Work out the finished part from the listing and answer in its coordinate system (mm). Round coordinates to 2 decimals unless told otherwise and drop trailing zeros. Order: outer loops, then holes, each group sorted by start corner. A loop starts at its lowest first (then second) coordinate and runs counter-clockwise, first axis right, second up. Notation, with made-up numbers: (89, -26.75) -> (128, -26.75) arc R23 cw to (128, 2.25) -> close; hole circle Ø11 at (70.25, 8). An arc over 180 degrees is marked (long way). Use a Markdown table: item, result. Add a question column.
Item 1: Flat-ended cylindrical pins translate along their axes: P1, Ø5, axis at y = -73, z = -9.5, coming from the +X side; P2, Ø2, axis at x = 0.5, z = -38.5, coming from the -Y side; P3, Ø2, axis at x = 2, y = -4.5, coming from the +Z side; P4, Ø4, axis at y = -60, z = -57.5, coming from the -X side. Find the tip coordinate at first contact, or state that the pin passes through.
Item 2: A cutting plane is placed at A-A, the plane y = -55. Determine the outline of the cut face in (x, z).
Item 3: A cutting plane is placed at D-D, the plane y = -72. Determine the outline of the cut face in (x, z), plus the area to 3 significant figures.
Item 4: A cutting plane is placed at C-C, the plane z = -47.9. Determine the outline of the cut face in (x, y) (3 decimals), plus the area to 3 significant figures.
Item 5: A cutting plane is placed at B-B, the plane x = 6. Determine the outline of the cut face in (y, z) (3 decimals), plus the area to 3 significant figures.
Item 6: Find the intervals of material crossed by L1, parallel to Z at x = 4.5, y = -12; L2, parallel to Y at x = 5, z = -47.9 (3 decimals); L3, parallel to Z at x = 7.75, y = -7 (3 decimals), in increasing order. Write a range as [from, to].
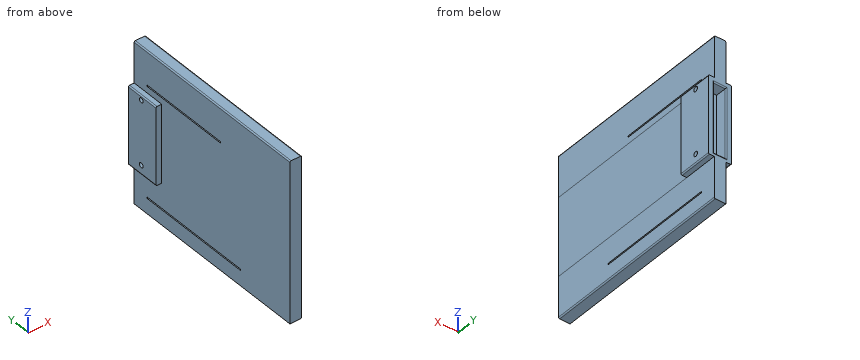
Autodesk Inventor part; units mm, degrees
ref_plane "YZ Plane" through (0, 0, 0) normal (1, 0, 0) x (0, 1, 0)
ref_plane "XZ Plane" through (0, 0, 0) normal (0, 1, 0) x (-1, 0, 0)
ref_plane "XY Plane" through (0, 0, 0) normal (0, 0, 1) x (1, 0, 0)
sketch "Sketch1" plane through (0, 0, 0) normal (1, 0, 0) x (0, 1, 0)
  line L0 (0, 0) -> (0, -70)
  line L1 (0, -70) -> (-85, -70)
  line L2 (-85, -70) -> (-85, 0)
  line L3 (-85, 0) -> (0, 0)
  dimension "d0" = 70
  dimension "d1" = 85
extrude "Extrusion1" add sketch "Sketch1" along normal blind 10
sketch "Sketch2" plane through (0, 0, 0) normal (0, 1, 0) x (1, 0, 0)
  line L0 (0, 0) -> (0, 70)
  line L1 (0, 0) -> (0, 20.125)
  line L2 (0, 20.125) -> (2.38, 20.125)
  line L3 (2.38, 20.125) -> (2.38, 50.375)
  line L4 (2.38, 50.375) -> (7.63, 50.375)
  line L5 (7.63, 50.375) -> (7.63, 20.125)
  line L6 (7.63, 20.125) -> (2.38, 20.125)
  dimension "d4" = 20.125
  dimension "d5" = 2.38
  dimension "d6" = 30.25
  dimension "d7" = 5.25
extrude "Extrusion2" cut sketch "Sketch2" against normal blind 5.1
sketch "Sketch3" plane through (0, 0, 0) normal (-1, 0, 0) x (0, 0, 1)
  line L0 (0, 0) -> (0, -85)
  line L1 (0, 0) -> (-20, 0)
  line L2 (-70, 0) -> (0, 0)
  line L3 (-20, 0) -> (-20, -7)
  circle A0 centre (-20, -7) radius 1.025
  circle A1 centre (-47.9, -7) radius 1.025
  line L4 (-20, -7) -> (-14.9, -7)
  line L5 (-14.9, -7) -> (-14.6, -7)
  line L6 (-14.6, -7) -> (-14.6, -47)
  line L7 (-14.6, -47) -> (-15.2, -47)
  line L8 (-15.2, -47) -> (-15.2, -7)
  line L9 (-15.2, -7) -> (-14.6, -7)
  line L10 (-20, -7) -> (-21.025, -7)
  line L11 (-46.875, -7) -> (-47.9, -7)
  line L12 (-47.9, -7) -> (-63.1, -7)
  line L13 (-63.1, -7) -> (-63.1, -47)
  line L14 (-63.1, -58) -> (-63.4, -58)
  line L15 (-63.4, -58) -> (-63.4, -7)
  line L16 (-63.4, -7) -> (-62.8, -7)
  line L17 (-62.8, -7) -> (-62.8, -58)
  line L18 (-62.8, -58) -> (-63.1, -58)
  line L19 (-47.9, -7) -> (-20, -7)
  line L20 (-63.1, -47) -> (-63.1, -58)
  line L21 (-70, -85) -> (-70, 0)
  line L22 (-63.1, -58) -> (-62.8, -58)
  line L23 (-62.8, -58) -> (-62.8, -7)
  line L24 (-63.4, -7) -> (-62.8, -7)
  dimension "d12" = 2.05
  dimension "d14" = 2.05
  dimension "d10" = 20
  dimension "d11" = 7
  dimension "d13" = 27.9
  dimension "d17" = 5.1
  dimension "d18" = 0.3
  dimension "d19" = 40
  dimension "d20" = 0.6
  dimension "d21" = 40
  dimension "d22" = 15.2
  dimension "d23" = 51
  dimension "d24" = 0.3
  dimension "d25" = 0.6
  dimension "d26" = 51
extrude "Extrusion3" cut sketch "Sketch3" against normal blind 10 contours A0 L4 L3 | A1 L12 L11 | L11 L12 A1 | L3 L10 A0 | L4 A0 L10
sketch "Sketch4" plane through (0, 0, 0) normal (-1, 0, 0) x (0, 0, 1)
  circle A0 centre (-19.9999, -6.9744) radius 1.25
  circle A1 centre (-47.8999, -6.9744) radius 1.25
  line L0 (-19.9999, -6.9744) -> (-14.8999, -6.9744)
  line L1 (-14.8999, -6.9744) -> (-14.5999, -6.9744)
  line L2 (-14.5999, -6.9744) -> (-14.5999, -46.9744)
  line L3 (-14.5999, -46.9744) -> (-15.1999, -46.9744)
  line L4 (-15.1999, -46.9744) -> (-15.1999, -6.9744)
  line L5 (-15.1999, -6.9744) -> (-14.5999, -6.9744)
  line L6 (-19.9999, -6.9744) -> (-21.2499, -6.9744)
  line L7 (-46.6499, -6.9744) -> (-47.8999, -6.9744)
  line L8 (-47.8999, -6.9744) -> (-63.0999, -6.9744)
  line L9 (-63.0999, -6.9744) -> (-63.0999, -46.9744)
  line L10 (-63.0999, -57.9744) -> (-63.3999, -57.9744)
  line L11 (-63.3999, -57.9744) -> (-63.3999, -6.9744)
  line L12 (-63.3999, -6.9744) -> (-62.7999, -6.9744)
  line L13 (-62.7999, -6.9744) -> (-62.7999, -57.9744)
  line L14 (-62.7999, -57.9744) -> (-63.0999, -57.9744)
  line L15 (-47.8999, -6.9744) -> (-19.9999, -6.9744)
  line L16 (-63.0999, -46.9744) -> (-63.0999, -57.9744)
  line L17 (-63.0999, -57.9744) -> (-62.7999, -57.9744)
  line L18 (-62.7999, -57.9744) -> (-62.7999, -6.9744)
  line L19 (-63.3999, -6.9744) -> (-62.7999, -6.9744)
  point P0 (0, 0)
  dimension "d27" = 2.5
  dimension "d29" = 2.5
  dimension "d28" = 27.9
  dimension "d30" = 5.1
  dimension "d31" = 0.3
  dimension "d32" = 40
  dimension "d33" = 0.6
  dimension "d34" = 40
  dimension "d35" = 15.2
  dimension "d36" = 51
  dimension "d37" = 0.3
  dimension "d38" = 0.6
  dimension "d39" = 51
extrude "Extrusion4" cut sketch "Sketch4" against normal blind 10 contours L13 L14 L16 L9 L8 | L0 L1 L2 L3 L4 | L9 L16 L10 L11 L12
sketch "Sketch5" plane through (0, 0, 0) normal (0, 1, 0) x (1, 0, 0)
  line L0 (0, 0) -> (10, 0)
  line L1 (0, 0) -> (2.5, 0)
  line L2 (2.5, 0) -> (2.5, 18)
  line L3 (2.5, 18) -> (0, 18)
  line L4 (0, 70) -> (0, 0)
  line L5 (10, 0) -> (7.5, 0)
  line L6 (7.5, 0) -> (7.5, 18)
  line L7 (7.5, 18) -> (10, 18)
  line L8 (10, 70) -> (10, 0)
  line L9 (10, 0) -> (10, 18)
  line L10 (7.5, 0) -> (7.5, 18)
  line L11 (10, 18) -> (10, 0)
  line L12 (0, 18.975) -> (10, 18.975)
  line L13 (10, 70) -> (10, 52)
  line L14 (10, 52) -> (7.5003, 52)
  line L15 (7.5003, 52) -> (7.5003, 70)
  line L16 (7.5003, 70) -> (10, 70)
  line L17 (10, 70) -> (10, 52)
  line L18 (10, 70) -> (10, 52)
  line L19 (0, 70) -> (0, 52)
  line L20 (0, 52) -> (2.5, 52)
  line L21 (2.5, 52) -> (2.5, 70)
  line L22 (2.5, 70) -> (0, 70)
  dimension "d42" = 2.5
  dimension "d43" = 18
  dimension "d44" = 2.5
  dimension "d45" = 18
  dimension "d46" = 18
  dimension "d47" = 18
extrude "Extrusion5" cut sketch "Sketch5" against normal through all contours L4 L3 L2 L0 | L4 L22 L21 L20 | L14 L15 L16 L8 | L6 L7 L8 L0
sketch "Sketch6" plane through (0, -85, -52) normal (0, -1, 0) x (1, 0, 0)
  line L0 (2.5, 34) -> (2.5, 52)
  line L1 (2.5, 0) -> (2.5, 34)
  line L2 (2.5, 34) -> (0, 34)
  line L3 (0, 0) -> (0, 34)
  line L4 (0, 34) -> (0, 0)
  line L5 (0, 0) -> (2.5, 0)
  line L6 (7.5003, 0) -> (7.5003, 34)
  line L7 (10.0003, 34) -> (10.0003, 0)
  line L8 (10.0003, 0) -> (7.5003, 0)
  line L9 (7.5003, -18) -> (7.5003, 0)
  line L10 (7.5, 52) -> (7.5, 34)
  line L11 (7.5, 34) -> (7.5, 4)
  line L12 (7.5, 4) -> (7.5003, 0)
  line L13 (7.5, 34) -> (10, 34)
  line L14 (7.5, 34) -> (10, 34)
  point P0 (0, 52)
  dimension "d52" = 2.5
  dimension "d53" = 30
extrude "Extrusion6" cut sketch "Sketch6" against normal blind 70 contours L5 L3 L2 L1
sketch "Sketch7" plane through (2.5, -85, -70) normal (0, -1, 0) x (1, 0, 0)
  line L0 (5, 52) -> (7.5, 52)
  line L1 (5.0003, 18) -> (5, 52)
  line L2 (5, 52) -> (7.5, 52)
  line L3 (7.5, 52) -> (7.5, 18)
  line L4 (7.5, 18) -> (5.0003, 18)
  point P0 (-2.5, 70)
extrude "Extrusion7" cut sketch "Sketch7" against normal blind 70
fillet "Fillet1" radius 0.5 11 edges at (7.5003, -42.5, -70) (2.5, -42.5, 0) (7.5, -42.5, 0) (10, -7.5, -18) (10, -7.5, -52) (0, -7.5, -18) (0, -7.5, -52) (7.63, 0, -35.25) (2.38, 0, -35.25) (5.005, 0, -20.125) (5.005, 0, -50.375)
properties part number "Chassis_Lower_Portion"
Reported:
| question | item | result |
|---|---|---|
| 1 | P1 | x = 7.5 |
| 1 | P2 | y = -15 |
| 1 | P3 | z = 0 |
| 1 | P4 | x = 2.5 |
| 2 | outline | (2.5, -70) -> (7, -70) arc R0.5 ccw to (7.5, -69.5) -> (7.5, -63.4) -> (2.5, -63.4) -> close; (2.5, -62.8) -> (7.5, -62.8) -> (7.5, -52) -> (7.5, -18) -> (7.5, -0.5) arc R0.5 ccw to (7, 0) -> (3, 0) arc R0.5 ccw to (2.5, -0.5) -> close |
| 3 | outline | (2.5, -70) -> (7, -70) arc R0.5 ccw to (7.5, -69.5) -> (7.5, -52) -> (7.5, -18) -> (7.5, -0.5) arc R0.5 ccw to (7, 0) -> (3, 0) arc R0.5 ccw to (2.5, -0.5) -> close |
| 3 | area | 350 mm² |
| 4 | outline | (0, -15) -> (2.5, -15) -> (2.5, -85) -> (7.5, -85) -> (7.5, -15) -> (10, -15) -> (10, -8.025) -> (0, -8.025) -> close; (0, -5.975) -> (10, -5.975) -> (10, 0) -> (8.13, 0) arc R0.5 ccw to (7.63, -0.5) -> (7.63, -5.1) -> (2.38, -5.1) -> (2.38, -0.5) arc R0.5 ccw to (1.88, 0) -> (0, 0) -> close |
| 4 | area | 453 mm² |
| 5 | outline | (-85, -70) -> (0, -70) -> (0, -50.875) arc R0.5 ccw to (-0.5, -50.375) -> (-5.1, -50.375) -> (-5.1, -20.125) -> (-0.5, -20.125) arc R0.5 ccw to (0, -19.625) -> (0, 0) -> (-85, 0) -> close; hole (-57.974, -63.4) -> (-6.974, -63.4) -> (-6.974, -62.8) -> (-57.974, -62.8) -> close; hole (-46.974, -15.2) -> (-6.974, -15.2) -> (-6.974, -14.6) -> (-46.974, -14.6) -> close; hole circle Ø2.05 at (-7, -47.9); hole circle Ø2.05 at (-7, -20) |
| 5 | area | 5,730 mm² |
| 6 | L1 | [-70, -63.4], [-62.8, -15.2], [-14.6, 0] |
| 6 | L2 | [-85, -8.025], [-5.975, -5.1] |
| 6 | L3 | [-52, -48.925], [-46.875, -21.025], [-18.975, -18] |
